Geometry: final body of the model. Coordinates: model frame, mm. Face numbers are marked on the shaded views. A direction names the side the tool comes from. Round coordinates to 2 decimals unless told otherwise and drop trailing zeros. Loops run counter-clockwise (first coordinate to the right, second up) from the corner with the lowest first, then second, coordinate; pieces in that order, holes last. Notation, with made-up numbers: (32, 39.5) - (80, 39.5) arc R16 ccw to (80, 49.5) - close; hole circle Ø4 at (24, -37.75). An arc over 180 degrees is marked (long way). Use CSV: the item, a comma, the result in double quotes.
from build123d import *

# Parameters (mm, degrees)
SKETCH1_W           = 65
SKETCH1_H           = 70
BOSS_EXTRUDE1_DEPTH = 76
CUT_EXTRUDE1_DEPTH  = 66
FILLET1_R           = 2
FILLET2_R           = 2


with BuildPart() as part:
    # Sketch1 → Boss-Extrude1 (new body)
    with BuildSketch(Plane(origin=(0, 0, 0), x_dir=(1, 0, 0), z_dir=(0, 1, 0))):
        with Locations((32.5, 35)):
            Rectangle(SKETCH1_W, SKETCH1_H)
    extrude(amount=BOSS_EXTRUDE1_DEPTH)

    # Sketch2 → Cut-Extrude1 (cut)
    with BuildSketch(Plane(origin=(0, 76, 0), x_dir=(1, 0, 0), z_dir=(0, 1, 0))):
        with BuildLine():
            Line((24.5, 0), (24.5, 25.395313644))
            ThreePointArc((24.5, 25.395313644), (32.5, 47.5), (40.5, 25.395313644))
            Line((40.5, 25.395313644), (40.5, 0))
            Line((40.5, 0), (24.5, 0))
        make_face()
    extrude(amount=-CUT_EXTRUDE1_DEPTH, mode=Mode.SUBTRACT)

    # Fillet1
    fillet1_edges = [part.edges().sort_by_distance(p)[0] for p in [
        (65, 76, -35),
        (52.75, 76, 0),
        (32.5, 76, -70),
        (24.5, 43, -25.395313644),
        (40.5, 43, -25.395313644),
        (40.5, 43, 0),
        (24.5, 43, 0),
        (32.5, 76, -47.5),
        (24.5, 76, -12.697656822),
        (40.5, 76, -12.697656822),
        (0, 76, -35),
        (32.5, 0, -70),
        (32.5, 0, 0),
        (0, 0, -35),
        (0, 38, -70),
        (65, 38, -70),
        (65, 38, 0),
        (0, 38, 0),
        (12.25, 76, 0),
    ]]
    fillet(fillet1_edges, radius=FILLET1_R)

    # Fillet2
    # the kernel refuses this fillet: 2 mm, written as the material it takes off along each edge
    with BuildSketch(Plane(origin=(63, 2, -68), x_dir=(1, 0, 0), z_dir=(0, -1, 0))) as fillet2_piece_1_section:
        Polygon((0, 0), (FILLET2_R, 0), (FILLET2_R, -FILLET2_R), (0, -FILLET2_R), align=None)
    fillet2_piece_1 = extrude(amount=FILLET2_R, mode=Mode.PRIVATE)
    fillet2_piece_1 = fillet2_piece_1 - Plane(origin=(63, 2, -68), x_dir=(-0.7071067811865475, 0, 0.7071067811865475), z_dir=(0, -1, 0)) * Sphere(FILLET2_R, mode=Mode.PRIVATE)
    add(fillet2_piece_1, mode=Mode.SUBTRACT)
    with BuildSketch(Plane(origin=(63, 2, -2), x_dir=(1, 0, 0), z_dir=(0, -1, 0))) as fillet2_piece_2_section:
        Polygon((0, 0), (FILLET2_R, 0), (FILLET2_R, FILLET2_R), (0, FILLET2_R), align=None)
    fillet2_piece_2 = extrude(amount=FILLET2_R, mode=Mode.PRIVATE)
    fillet2_piece_2 = fillet2_piece_2 - Plane(origin=(63, 2, -2), x_dir=(-0.7071067811865475, 0, -0.7071067811865475), z_dir=(0, -1, 0)) * Sphere(FILLET2_R, mode=Mode.PRIVATE)
    add(fillet2_piece_2, mode=Mode.SUBTRACT)
    with BuildSketch(Plane(origin=(65, 0, -2), x_dir=(-1, 0, 0), z_dir=(0, 0, -1))) as fillet2_piece_3:
        with BuildLine():
            CenterArc((FILLET2_R, FILLET2_R), FILLET2_R, 180, 90)
            Line((0, FILLET2_R), (0, 0))
            Line((0, 0), (FILLET2_R, 0))
        make_face()
    extrude(amount=66, mode=Mode.SUBTRACT)


solid = part.part
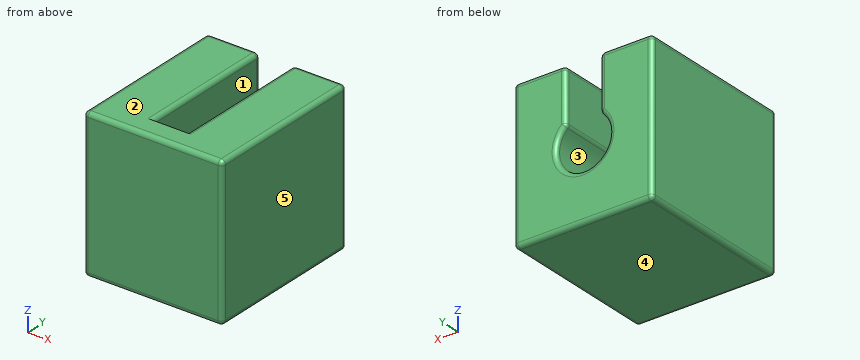
Item 1: Section B-B on x = 32.5. Return the cut outline in (y, z).
Final values:
outline,"(0, -68) arc R2 ccw to (2, -70) - (74, -70) arc R2 ccw to (76, -68) - (76, -49.5) arc R2 ccw to (74, -47.5) - (10, -47.5) - (10, 0) - (2, 0) arc R2 ccw to (0, -2) - close"
Item 2: Material intervals for line 1 (X direction, y = 45, z = -35); line 2 (X direction, y = 31.5, z = -6); line 3 (Z direction, x = 32.5, y = 42.5), sorted ascending.
Final values:
line 1,"x = 0 to 20, 45 to 65"
line 2,"x = 0 to 24.5, 40.5 to 65"
line 3,"z = -70 to -47.5"
Item 3: Reachability of the marked faces 1 and 2 from +Z, -Z, +X, -X, +Y, -Y: full face, straight path, thin tool, end or side. Return the list, or none.
Final values:
face 1,"+Z, +Y"
face 2,"+Z, +X, -X, +Y, -Y"
Item 4: Mould query, pull axis X, two halves, no side actions, for the marked faces 3, 4 and 5. Classes: released by +X, released by -X, zero draft, split by the parting line, or undercut.
Final values:
face 3,"undercut"
face 4,"zero draft"
face 5,"released by +X"
Item 5: Pin query (flat end, axial travel): P1, Ø15, axis at x = 32.5, z = -35, coming from the +Y side. Return the tip coordinate at first contact, or that it passes through.
Final values:
P1,"stops at y = 10"
Item 6: Section A-A on y = 71. Return the cut outline in (x, z), plus the area to 3 significant figures.
Final values:
outline,"(0, -68) arc R2 ccw to (2, -70) - (63, -70) arc R2 ccw to (65, -68) - (65, -2) arc R2 ccw to (63, 0) - (42.5, 0) arc R2 ccw to (40.5, -2) - (40.5, -24.5) arc R2 ccw to (41.12, -25.95) arc R12.5 cw (long way) to (23.88, -25.95) arc R2 ccw to (24.5, -24.5) - (24.5, -2) arc R2 ccw to (22.5, 0) - (2, 0) arc R2 ccw to (0, -2) - close"
area,"3,680 mm²"
Item 7: Section C-C on z = -11.5. Return the cut outline in (x, y).
Final values:
outline,"(0, 2) arc R2 ccw to (2, 0) - (63, 0) arc R2 ccw to (65, 2) - (65, 74) arc R2 ccw to (63, 76) - (42.5, 76) arc R2 ccw to (40.5, 74) - (40.5, 10) - (24.5, 10) - (24.5, 74) arc R2 ccw to (22.5, 76) - (2, 76) arc R2 ccw to (0, 74) - close"
